from build123d import *

# Parameters (mm, degrees)
BOSS_EXTRUDE1_DEPTH                           = 3.175
FILLET1_R                                     = 12.7
CUT_EXTRUDE1_DEPTH                            = 4.175
CSK_FOR_8_FLAT_HEAD_MACHINE_SCREW1_AT_2_COUNT = 2
CSK_FOR_8_FLAT_HEAD_MACHINE_SCREW1_AT_2_PITCH = 41.643335968
CSK_FOR_8_FLAT_HEAD_MACHINE_SCREW1_AT_3_COUNT = 2
CSK_FOR_8_FLAT_HEAD_MACHINE_SCREW1_AT_3_PITCH = 55.434622241
CSK_FOR_8_FLAT_HEAD_MACHINE_SCREW1_AT_4_COUNT = 2
CSK_FOR_8_FLAT_HEAD_MACHINE_SCREW1_AT_4_PITCH = 50.008853946
CSK_FOR_8_FLAT_HEAD_MACHINE_SCREW1_AT_5_COUNT = 2
CSK_FOR_8_FLAT_HEAD_MACHINE_SCREW1_AT_5_PITCH = 82.918335968
CSK_FOR_8_FLAT_HEAD_MACHINE_SCREW1_AT_6_COUNT = 2
CSK_FOR_8_FLAT_HEAD_MACHINE_SCREW1_AT_6_PITCH = 86.127052655
CSK_FOR_8_FLAT_HEAD_MACHINE_SCREW1_AT_7_COUNT = 2
CSK_FOR_8_FLAT_HEAD_MACHINE_SCREW1_AT_7_PITCH = 138.300491667
CUT_EXTRUDE2_REACH                            = 5.175
SKETCH5_R                                     = 5.55625


with BuildPart() as part:
    # Sketch1 → Boss-Extrude1 (new body)
    with BuildSketch(Plane.XY):
        Polygon((-234.752967181, 12.7), (-91.997327393, 12.7), (-91.997327393, -7.416979032), (-74.533465131, -7.416979032), (-50.700252483, -210.6746006), (-234.752967181, -270.542758328), align=None)
    extrude(amount=BOSS_EXTRUDE1_DEPTH)

    # Fillet1
    fillet1_edges = [part.edges().sort_by_distance(p)[0] for p in [
        (-74.533465131, -7.416979032, 1.5875),
        (-50.700252483, -210.6746006, 1.5875),
    ]]
    fillet(fillet1_edges, radius=FILLET1_R)

    # Sketch2 → Cut-Extrude1 (cut, through all)
    with BuildSketch(Plane.XY.offset(3.175)):
        Polygon((-234.752967181, -270.542758328), (-222.67581909, -266.614337017), (-234.752967181, -229.485553098), align=None)
    extrude(amount=-CUT_EXTRUDE1_DEPTH, mode=Mode.SUBTRACT)

    # Sketch4 → CSK for #8 Flat Head Machine Screw1 (revolve, cut)
    with BuildSketch(Plane(origin=(-203.96982343, -247.917009556, 0), x_dir=(0, 1, 0), z_dir=(1, 0, 0))):
        Polygon((0, 0), (0, 3.175), (2.45745, 3.175), (2.45745, 2.02344051), (4.2164, 0), align=None)
    csk_for_8_flat_head_machine_screw1 = revolve(axis=Axis((-203.96982343, -247.917009556, -6.35), (0, 0, 1)), mode=Mode.SUBTRACT)

    # CSK for #8 Flat Head Machine Screw1 at 2: CSK for #8 Flat Head Machine Screw1 ×2
    with Locations(*[Vector(0.950956543, 0.309324513, 0) * (i * CSK_FOR_8_FLAT_HEAD_MACHINE_SCREW1_AT_2_PITCH) for i in range(1, CSK_FOR_8_FLAT_HEAD_MACHINE_SCREW1_AT_2_COUNT)]):
        add(csk_for_8_flat_head_machine_screw1, mode=Mode.SUBTRACT)

    # CSK for #8 Flat Head Machine Screw1 at 3: CSK for #8 Flat Head Machine Screw1 ×2
    with Locations(*[Vector(0.510201208, 0.860055072, 0) * (i * CSK_FOR_8_FLAT_HEAD_MACHINE_SCREW1_AT_3_PITCH) for i in range(1, CSK_FOR_8_FLAT_HEAD_MACHINE_SCREW1_AT_3_COUNT)]):
        add(csk_for_8_flat_head_machine_screw1, mode=Mode.SUBTRACT)

    # CSK for #8 Flat Head Machine Screw1 at 4: CSK for #8 Flat Head Machine Screw1 ×2
    with Locations(*[Vector(-0.309324513, 0.950956543, 0) * (i * CSK_FOR_8_FLAT_HEAD_MACHINE_SCREW1_AT_4_PITCH) for i in range(1, CSK_FOR_8_FLAT_HEAD_MACHINE_SCREW1_AT_4_COUNT)]):
        add(csk_for_8_flat_head_machine_screw1, mode=Mode.SUBTRACT)

    # CSK for #8 Flat Head Machine Screw1 at 5: CSK for #8 Flat Head Machine Screw1 ×2
    with Locations(*[Vector(0.950956543, 0.309324513, 0) * (i * CSK_FOR_8_FLAT_HEAD_MACHINE_SCREW1_AT_5_PITCH) for i in range(1, CSK_FOR_8_FLAT_HEAD_MACHINE_SCREW1_AT_5_COUNT)]):
        add(csk_for_8_flat_head_machine_screw1, mode=Mode.SUBTRACT)

    # CSK for #8 Flat Head Machine Screw1 at 6: CSK for #8 Flat Head Machine Screw1 ×2
    with Locations(*[Vector(0.83188266, 0.554951566, 0) * (i * CSK_FOR_8_FLAT_HEAD_MACHINE_SCREW1_AT_6_PITCH) for i in range(1, CSK_FOR_8_FLAT_HEAD_MACHINE_SCREW1_AT_6_COUNT)]):
        add(csk_for_8_flat_head_machine_screw1, mode=Mode.SUBTRACT)

    # CSK for #8 Flat Head Machine Screw1 at 7: CSK for #8 Flat Head Machine Screw1 ×2
    with Locations(*[Vector(0.950956543, 0.309324513, 0) * (i * CSK_FOR_8_FLAT_HEAD_MACHINE_SCREW1_AT_7_PITCH) for i in range(1, CSK_FOR_8_FLAT_HEAD_MACHINE_SCREW1_AT_7_COUNT)]):
        add(csk_for_8_flat_head_machine_screw1, mode=Mode.SUBTRACT)

    # Sketch5 → Cut-Extrude2 (cut, up to next)
    with BuildSketch(Plane.XY.offset(3.175), mode=Mode.PRIVATE) as cut_extrude2_sk1:
        with Locations((-90.146601991, -37.840751583)):
            Circle(SKETCH5_R)
    cut_extrude2_tool1 = extrude(cut_extrude2_sk1.sketch, amount=-CUT_EXTRUDE2_REACH, mode=Mode.PRIVATE) & part.part
    add(cut_extrude2_tool1.solids().sort_by_distance((-90.146602, -37.840752, 3.175))[0], mode=Mode.SUBTRACT)
    # Sketch5 → Cut-Extrude2 (cut, up to next)
    with BuildSketch(Plane.XY.offset(3.175), mode=Mode.PRIVATE) as cut_extrude2_sk2:
        with Locations((-75.576674395, -162.097975039)):
            Circle(SKETCH5_R)
    cut_extrude2_tool2 = extrude(cut_extrude2_sk2.sketch, amount=-CUT_EXTRUDE2_REACH, mode=Mode.PRIVATE) & part.part
    add(cut_extrude2_tool2.solids().sort_by_distance((-75.576674, -162.097975, 3.175))[0], mode=Mode.SUBTRACT)


solid = part.part
Geometry check sheet. Reference: the model listing, model coordinates, mm. Round coordinates to 2 decimals unless told otherwise and drop trailing zeros. Order: outer loops, then holes, each group sorted by start corner. A loop starts at its lowest first (then second) coordinate and runs counter-clockwise, first axis right, second up. Notation, with made-up numbers: (-32.5, 73.25) - (-12.5, 73.25) arc R36 ccw to (-12.5, 109.25) - close; hole circle Ø3 at (48, -20). An arc over 180 degrees is marked (long way). One line per question, with ' | ' between items. Start each with the question number.
(1) Sectioned sample at B-B on x = -154. Record the cut outline in (y, z) (3 decimals), and give its area (3 significant figures).
(2) Release check for a two-part mould opening along X. For faces 1 (the cylindrical face through (-85.014, -39.969, 1.61)), 2 (the flat face through (-228.63, -248.31, 1.61)), 3 (the conical face through (-162.81, -237.07, 1.9)), 4 (the cylindrical face through (-53.767, -208.565, 1.61)) record: released by +X, released by -X, zero draft, split by the parting line, or undercut.
(3) Sectioned sample at C-C on y = -81. Record the cut outline in (x, z) (3 decimals).
(4) Sectioned sample at A-A on z = 1.1. Count the separate pieces of the cut face and the enclosed holes in it, and give its area (3 significant figures).
(5) Thickness scan on L1, parallel to X at y = -199, z = 0.5; L2, parallel to Y at x = -77, z = 0.45; L3, parallel to Y at x = -220.5, z = 1.45. Record the ranges inside material, lowest first. Write a range as [from, to].
(6) Depth check by flat-ended pin: pin 1 Ø14.5 at (x, y) = (-75.58, -162.1) entering from -Z; pin 2 Ø5.5 at (x, y) = (-203.97, -247.92) entering from -Z; pin 3 Ø8 at (x, y) = (-132.32, -200.12) entering from -Z; pin 4 Ø1.6 at (x, z) = (-89, 1.5) entering from +Y. Enter the tip coordinate at first touch or a pass-through.
Conclusion:
1) outline: (-244.276, 0) - (12.7, 0) - (12.7, 3.175) - (-244.276, 3.175) - close | area: 816 mm2
2) face 1: undercut | face 2: released by -X | face 3: undercut | face 4: released by +X
3) outline: (-234.753, 0) - (-65.905, 0) - (-65.905, 3.175) - (-234.753, 3.175) - close
4) separate pieces: 1 | enclosed holes: 9 | area: 42,600 mm2
5) L1: x = [-234.75, -222.97], [-215.91, -179.26], [-172.11, -135.93], [-128.71, -52.07] | L2: y = [-219.23, -167.47], [-156.73, -10.99] | L3: y = [-265.91, -203.12], [-197.6, 12.7]
6) pin 1: stops at z = 0 | pin 2: stops at z = 1.68 | pin 3: stops at z = 0.25 | pin 4: stops at y = -7.42
